Input: dimensioned drawing with shaded views. Units: mm. Origin: part minimum x, y, z. A direction names the side the tool comes from. Give positions to 0.01 mm unless a question says otherwise; leave off trailing zeros. Write each loop counter-clockwise with the first axis right and the second up, starting at its lowest first coordinate (ties: lowest second). Pieces come first, ordered by that corner, then holes. Notation, with made-up numbers: (63.25, -1) -> (113.25, -1) arc R22 ccw to (113.25, 22) -> close; hole circle Ø11 at (-9, 87.25). An arc over 180 degrees is marked (long way). Answer as a JSON object with one key per item and string values. Group by question number.
(1) Section query A-A on z = 4. Output: boundary loops of the cut face in (x, y), plus the area to 3 significant figures.
(2) Section query C-C on x = 8.5. Output: boundary loops of the cut face in (y, z).
(3) Section query B-B on y = 6.5. Output: boundary loops of the cut face in (x, z), plus the area to 3 significant figures.
(4) Material intervals for probe 1 along Y at (x, z) = (16, 2); probe 2 along X at (y, z) = (13.25, 9.75), sorted ascending.
(5) Set-up query: the marked faces 1 and 2. Return all of +Z, -Z, +X, -X, +Y, -Y with unobstructed straight access to the full face (end or side cutting, diameter ignored); none if empty.
(6) Draft query along X for the marked faces 3, 4 and 5. Return one class per face: +X half, -X half, draft (parallel to the pull), parting line (faces both ways), or undercut.
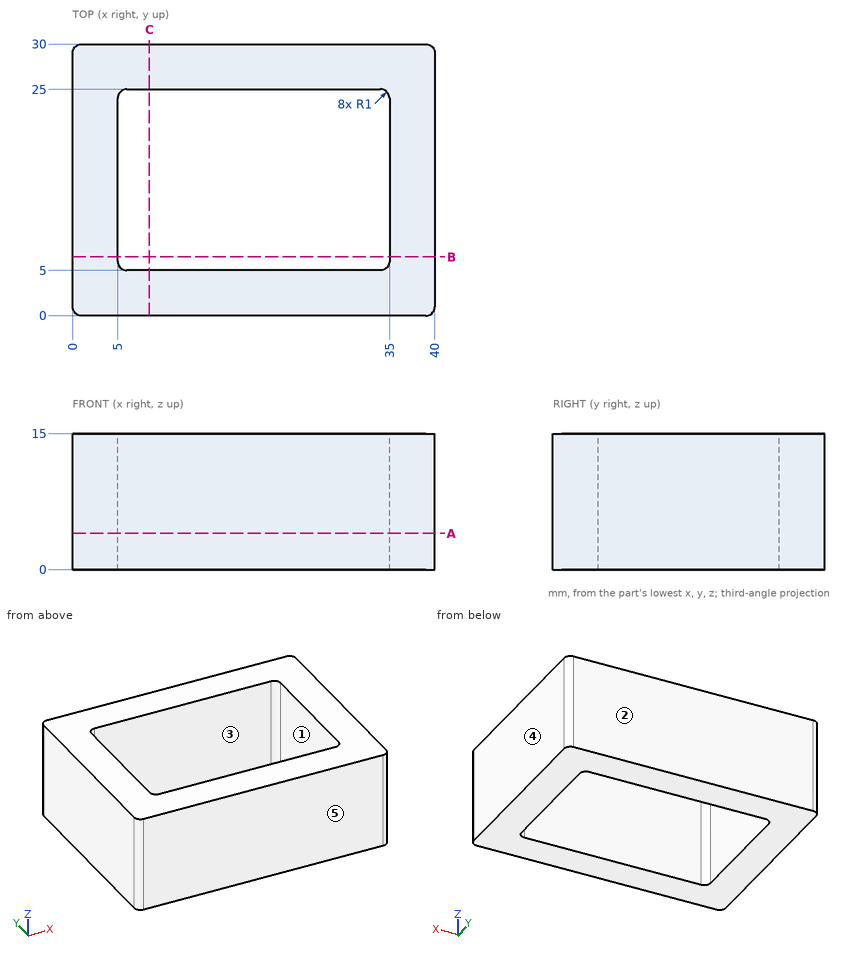
Answer list:
{
 "1": {"outline": "(0, 1) arc R1 ccw to (1, 0) -> (39, 0) arc R1 ccw to (40, 1) -> (40, 29) arc R1 ccw to (39, 30) -> (1, 30) arc R1 ccw to (0, 29) -> close; hole (5, 6) arc R1 ccw to (6, 5) -> (34, 5) arc R1 ccw to (35, 6) -> (35, 24) arc R1 ccw to (34, 25) -> (6, 25) arc R1 ccw to (5, 24) -> close", "area": "600 mm2"},
 "2": {"outline": "(0, 0) -> (5, 0) -> (5, 15) -> (0, 15) -> close; (25, 0) -> (30, 0) -> (30, 15) -> (25, 15) -> close"},
 "3": {"outline": "(0, 0) -> (5, 0) -> (5, 15) -> (0, 15) -> close; (35, 0) -> (40, 0) -> (40, 15) -> (35, 15) -> close", "area": "150 mm2"},
 "4": {"probe 1": "0 to 5, 25 to 30", "probe 2": "0 to 5, 35 to 40"},
 "5": {"face 1": "+Z, -Z", "face 2": "+Z, -Z, +X, -X, +Y"},
 "6": {"face 3": "undercut", "face 4": "+X half", "face 5": "draft"}
}
